Could you check a few things on this model? Use its own coordinates, in mm. Round coordinates to 2 decimals unless told otherwise and drop trailing zeros. Order: outer loops, then holes, each group sorted by start corner. A loop starts at its lowest first (then second) coordinate and runs counter-clockwise, first axis right, second up. Notation, with made-up numbers: (78.5, 6) -> (89.5, 6) arc R33 cw to (89.5, 40) -> close; hole circle Ø5 at (-11.75, -33). An arc over 180 degrees is marked (long way). One line per question, with ' | ' between items.
```python
from build123d import *

# Parameters (mm, degrees)
ESQUISSE1_R             = 37.5
ESQUISSE1_R_2           = 9.75
BOSS_EXTRU_1_DEPTH      = 24
CONG_1_R                = 10
ESQUISSE3_W             = 3
ESQUISSE3_H             = 4
ENL_V_MAT_EXTRU_1_DEPTH = 59.210823736


with BuildPart() as part:
    # Esquisse1 → Boss.-Extru.1 (new body)
    with BuildSketch(Plane.XY):
        Circle(ESQUISSE1_R)
        Circle(ESQUISSE1_R_2, mode=Mode.SUBTRACT)
    extrude(amount=BOSS_EXTRU_1_DEPTH)

    # Congé1
    cong_1_edges = [part.edges().sort_by_distance(p)[0] for p in [
        (-37.5, 0, 0),
        (-37.5, 0, 24),
    ]]
    fillet(cong_1_edges, radius=CONG_1_R)

    # Esquisse3 → Enlèv. mat.-Extru.1 (cut, through all)
    with BuildSketch(Plane.XY.offset(24)):
        Polygon((15.228907027, 6.525365182), (16.15595801, 3.672195633), (12.351731945, 2.436127655), (11.424680962, 5.289297204), align=None)
        with Locations((0, 14.5)):
            Rectangle(ESQUISSE3_W, ESQUISSE3_H)
        Polygon((10.911982154, -12.467102529), (8.484931171, -14.230458286), (6.133790162, -10.994390308), (8.560841145, -9.231034551), align=None)
        Polygon((-8.484931171, -14.230458286), (-10.911982154, -12.467102529), (-8.560841145, -9.231034551), (-6.133790162, -10.994390308), align=None)
        Polygon((-16.15595801, 3.672195633), (-15.228907027, 6.525365182), (-11.424680962, 5.289297204), (-12.351731945, 2.436127655), align=None)
    extrude(amount=-ENL_V_MAT_EXTRU_1_DEPTH, mode=Mode.SUBTRACT)


solid = part.part
```
1. I want a section at C-C on x = 0. List the corners of the cut face in (y, z) for me.
From the geometry:
outline: (-37.5, 10) arc R10 ccw to (-27.5, 0) -> (-9.75, 0) -> (-9.75, 24) -> (-27.5, 24) arc R10 ccw to (-37.5, 14) -> close; (9.75, 0) -> (12.5, 0) -> (12.5, 24) -> (9.75, 24) -> close; (16.5, 0) -> (27.5, 0) arc R10 ccw to (37.5, 10) -> (37.5, 14) arc R10 ccw to (27.5, 24) -> (16.5, 24) -> close
2. I need wall thicknesses on probe 1 along Y at (x, z) = (0, 11.25); probe 2 along X at (y, z) = (-10.5, 3); probe 3 along Y at (x, z) = (0, 16.25). Which ranges of each line are inside material? Lowest first, please.
From the geometry:
probe 1: y = -37.5 to -9.75, 9.75 to 12.5, 16.5 to 37.5 | probe 2: x = -33.01 to -9.48, -6.81 to 6.81, 9.48 to 33.01 | probe 3: y = -37.24 to -9.75, 9.75 to 12.5, 16.5 to 37.24
3. I want a section at B-B on z = 11.25. List the corners of the cut face in (x, y) for me, and give its area (3 significant figures).
From the geometry:
outline: circle Ø75 at (0, 0); hole (-16.16, 3.67) -> (-12.35, 2.44) -> (-11.42, 5.29) -> (-15.23, 6.53) -> close; hole (-10.91, -12.47) -> (-8.48, -14.23) -> (-6.13, -10.99) -> (-8.56, -9.23) -> close; hole circle Ø19.5 at (0, 0); hole (-1.5, 12.5) -> (1.5, 12.5) -> (1.5, 16.5) -> (-1.5, 16.5) -> close; hole (6.13, -10.99) -> (8.48, -14.23) -> (10.91, -12.47) -> (8.56, -9.23) -> close; hole (11.42, 5.29) -> (12.35, 2.44) -> (16.16, 3.67) -> (15.23, 6.53) -> close | area: 4,060 mm²
4. I want a section at A-A on y = 0. List the corners of the cut face in (x, z) for me, and give its area (3 significant figures).
From the geometry:
outline: (-37.5, 10) arc R10 ccw to (-27.5, 0) -> (-9.75, 0) -> (-9.75, 24) -> (-27.5, 24) arc R10 ccw to (-37.5, 14) -> close; (9.75, 0) -> (27.5, 0) arc R10 ccw to (37.5, 10) -> (37.5, 14) arc R10 ccw to (27.5, 24) -> (9.75, 24) -> close | area: 1,250 mm²
5. I'm going to push flat-ended pins straight in: pin 1 (5 mm diameter, centred on y = 15, z = 12, fed in from -X); pin 2 (2 mm diameter, centred on y = -3, z = 15.5, fed in from +X); pin 3 (4.5 mm diameter, centred on y = 14.5, z = 15.5, fed in from +X). Where does each tip first touch, or does it pass through?
From the geometry:
pin 1: stops at x = -35.36 | pin 2: stops at x = 37.4 | pin 3: stops at x = 35.37
